```python
from build123d import *

# Parameters (mm, degrees)
F0_R     = 139.7
F0_R_2   = 11.1125
F0_R_3   = 76.2
F1_DEPTH = 23.876
F2_R     = 101.6
F2_R_2   = 76.2
F3_DEPTH = 3.175
F4_R     = 1.905


with BuildPart() as f1:
    # F0 (on Front) → F1 (new body)
    with BuildSketch(Plane.XZ):
        Circle(F0_R)
        with Locations((-46.170756, -111.466066)):
            Circle(F0_R_2, mode=Mode.SUBTRACT)
        with Locations((-111.466066, -46.170756)):
            Circle(F0_R_2, mode=Mode.SUBTRACT)
        with Locations((46.170756, -111.466066)):
            Circle(F0_R_2, mode=Mode.SUBTRACT)
        with Locations((111.466066, -46.170756)):
            Circle(F0_R_2, mode=Mode.SUBTRACT)
        with Locations((-111.466066, 46.170756)):
            Circle(F0_R_2, mode=Mode.SUBTRACT)
        with Locations((-46.170756, 111.466066)):
            Circle(F0_R_2, mode=Mode.SUBTRACT)
        Circle(F0_R_3, mode=Mode.SUBTRACT)
        with Locations((111.466066, 46.170756)):
            Circle(F0_R_2, mode=Mode.SUBTRACT)
        with Locations((46.170756, 111.466066)):
            Circle(F0_R_2, mode=Mode.SUBTRACT)
    extrude(amount=F1_DEPTH)

    # F2 (on face) → F3 (join)
    with BuildSketch(Plane.XZ.offset(23.876)):
        Circle(F2_R)
        Circle(F2_R_2, mode=Mode.SUBTRACT)
    extrude(amount=F3_DEPTH)

    # F4
    f4_edges = [f1.edges().sort_by_distance(p)[0] for p in [
        (-139.7, 0, 0),
        (-139.7, -23.876, 0),
        (-101.6, -23.876, 0),
    ]]
    fillet(f4_edges, radius=F4_R)


solid = f1.part
```
Work out the finished part from the listing and answer in its coordinate system (mm). A direction names the side the tool comes from. Round coordinates to 2 decimals unless told otherwise and drop trailing zeros. Loops run counter-clockwise (first coordinate to the right, second up) from the corner with the lowest first, then second, coordinate; pieces in that order, holes last. Notation, with made-up numbers: (82.25, -12) -> (88.25, -12) arc R19 ccw to (88.25, -7) -> close; hole circle Ø5 at (88.25, 69.25). An arc over 180 degrees is marked (long way). Write each question's results on one line, items separated by ' | '. Start each with the question number.
1. A tool of negligible diameter and unlimited length cuts with its end or side. For faces 1 (the face through (103.276, -11.771, 53.681)), 2 (the face through (30, -23.876, -101)), from which of +Z, -Z, +X, -X, +Y, -Y can it reach the whole face along a straight path? Write none if from no direction.
2. Section A-A (z = 0) is taken. Determine the outline of the cut face in (x, y) (3 decimals), plus the area to 3 significant figures.
3. Section B-B (x = 0) is taken. Determine the outline of the cut face in (y, z) (3 decimals).
4. Section C-C (y = -12) is taken. State how many separate pieces and enclosed holes the cut face has, plus the area to 3 significant figures.
5. Find the intervals of material crossed by probe 1 along X at (y, z) = (-12.5, -104.5); probe 2 along Z at (x, y) = (-49, -23); probe 3 along Z at (x, y) = (-103.5, -10.75), in increasing order. Write a range as from..to.
6. Given pin 1 Ø8 at (y, z) = (-5, 83) entering from +X; pin 2 Ø10 at (y, z) = (-15.5, 96.5) entering from +X; pin 3 Ø3 at (y, z) = (-21, -51.5) entering from +X, each flat-ended and moving along its own axis, determine where each tip first touches the part or whether it passes through.
Evaluation:
1) face 1: +Y, -Y | face 2: -Y
2) outline: (-139.7, -21.971) arc R1.905 ccw to (-137.795, -23.876) -> (-103.505, -23.876) arc R1.905 cw to (-101.6, -25.781) -> (-101.6, -27.051) -> (-76.2, -27.051) -> (-76.2, 0) -> (-137.795, 0) arc R1.905 ccw to (-139.7, -1.905) -> close; (76.2, -27.051) -> (101.6, -27.051) -> (101.6, -25.781) arc R1.905 cw to (103.505, -23.876) -> (137.795, -23.876) arc R1.905 ccw to (139.7, -21.971) -> (139.7, -1.905) arc R1.905 ccw to (137.795, 0) -> (76.2, 0) -> close | area: 3,190 mm2
3) outline: (-27.051, -101.6) -> (-25.781, -101.6) arc R1.905 cw to (-23.876, -103.505) -> (-23.876, -137.795) arc R1.905 ccw to (-21.971, -139.7) -> (-1.905, -139.7) arc R1.905 ccw to (0, -137.795) -> (0, -76.2) -> (-27.051, -76.2) -> close; (-27.051, 76.2) -> (0, 76.2) -> (0, 137.795) arc R1.905 ccw to (-1.905, 139.7) -> (-21.971, 139.7) arc R1.905 ccw to (-23.876, 137.795) -> (-23.876, 103.505) arc R1.905 cw to (-25.781, 101.6) -> (-27.051, 101.6) -> close
4) separate pieces: 1 | enclosed holes: 9 | area: 40,000 mm2
5) probe 1: x = -92.71..-54.83, -37.51..37.51, 54.83..92.71 | probe 2: z = -130.5..-122.21, -100.72..-58.36, 58.36..100.72, 122.21..130.5 | probe 3: z = -93.83..-53.92, -38.42..38.42, 53.92..93.83
6) pin 1: stops at x = 115.22 | pin 2: stops at x = 105.56 | pin 3: stops at x = 130.45
